from build123d import *

# Parameters (mm, degrees)
F1_DEPTH = 3.175


with BuildPart() as f1:
    # F0 (on Front) → F1 (new body)
    with BuildSketch(Plane.XZ):
        with BuildLine():
            Line((0, 152.4), (0, 0))
            Line((0, 0), (139.7, 0))
            Line((139.7, 0), (292.1, 234.176429))
            Line((292.1, 234.176429), (596.9, 234.176429))
            Line((596.9, 234.176429), (749.3, 0))
            Line((749.3, 0), (1943.1, 0))
            Line((1943.1, 0), (1943.1, 304.8))
            ThreePointArc((1943.1, 304.8), (1920.781537, 358.681537), (1866.9, 381))
            Line((1866.9, 381), (101.6, 381))
            Line((101.6, 381), (0, 152.4))
        make_face()
    extrude(amount=F1_DEPTH)


solid = f1.part
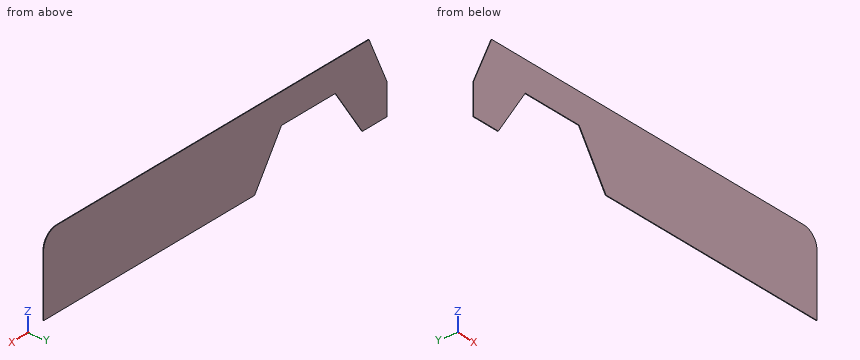
Design review of the part built by this model. Coordinates are the model's own, in mm. Give positions to 0.01 mm unless a question says otherwise; leave off trailing zeros. Loops run counter-clockwise (first coordinate to the right, second up) from the corner with the lowest first, then second, coordinate; pieces in that order, holes last. Notation, with made-up numbers: M 6.5,4.5 L 49.5,4.5 A27 ccw 49.5,33.5 Z; hole C 81,5 d2. An arc over 180 degrees is marked long. One line per question, with ' | ' between items. Start each with the question number.
1. Add section D-D (x = 334). Write out the cut boundary in (y, z) (3 decimals), plus the area to 3 significant figures.
2. Add section A-A (y = -1.1). Write out the cut boundary in (x, z), plus the area to 3 significant figures.
3. Add section B-B (z = 211). Write out the cut boundary in (x, y) (3 decimals).
4. Add section C-C (z = 42). Write out the cut boundary in (x, y) (3 decimals), plus the area to 3 significant figures.
5. Insertion check: P1, Ø1, axis at x = 436, y = -1.5, coming from the -Z side. The pin has a flat end and moves straight along its axis. Give the tip position at first contact, or say it passes through.
6. To check wall thickness, follow L1, parallel to X at y = -2.3, z = 41; L2, parallel to X at y = -3, z = 148; L3, parallel to Z at x = 554, y = -2.45. State the ranges of each line that lie inside material, in increasing order.
Worked out:
1) outline: M -3.175,234.176 L 0,234.176 L 0,381 L -3.175,381 Z | area: 466 mm²
2) outline: M 0,0 L 139.7,0 L 292.1,234.18 L 596.9,234.18 L 749.3,0 L 1943.1,0 L 1943.1,304.8 A76.2 ccw 1866.9,381 L 101.6,381 L 0,152.4 Z | area: 620,000 mm²
3) outline: M 26.044,-3.175 L 277.017,-3.175 L 277.017,0 L 26.044,0 Z; M 611.983,-3.175 L 1943.1,-3.175 L 1943.1,0 L 611.983,0 Z
4) outline: M 0,-3.175 L 167.033,-3.175 L 167.033,0 L 0,0 Z; M 721.967,-3.175 L 1943.1,-3.175 L 1943.1,0 L 721.967,0 Z | area: 4,410 mm²
5) P1: stops at z = 234.18
6) L1: x = 0 to 166.38, 722.62 to 1943.1 | L2: x = 0 to 236.02, 652.98 to 1943.1 | L3: z = 234.18 to 381
